```python
from build123d import *

# Parameters (mm, degrees)
EXTRUDE_1_DEPTH     = 20
EXTRUDE_2_DEPTH     = 20
CUT_EXTRUDE_1_DEPTH = 15
SCALE_1_SCALE       = 0.2


with BuildPart() as part:
    # 草圖1 → 填料-伸長1 (new body)
    with BuildSketch(Plane(origin=(0, 0, 0), x_dir=(1, 0, 0), z_dir=(0, 1, 0))):
        Polygon((-5, 5), (-5, -10), (15, -5), (15, 5), align=None)
    extrude(amount=EXTRUDE_1_DEPTH)

    # 草圖1<3> → 填料-伸長2 (add)
    with BuildSketch(Plane(origin=(0, 0, 0), x_dir=(1, 0, 0), z_dir=(0, 1, 0))):
        Polygon((-15, -10), (-5, -10), (-5, 5), (15, 5), (15, 10), (-15, 10), align=None)
    extrude(amount=EXTRUDE_2_DEPTH)

    # 草圖2 → 除料-伸長1 (cut)
    with BuildSketch(Plane.XY.offset(10)):
        Polygon((-5, 20), (15, 5), (15, 20), align=None)
    extrude(amount=-CUT_EXTRUDE_1_DEPTH, mode=Mode.SUBTRACT)


with BuildPart() as part_1:
    # 縮放比例1: scaled about (-2.387387387, 9.02027027, -1.06981982)
    add(part.part.scale(SCALE_1_SCALE).moved(Location((-1.90990991, 7.216216216, -0.855855856))))


solid = part_1.part
```
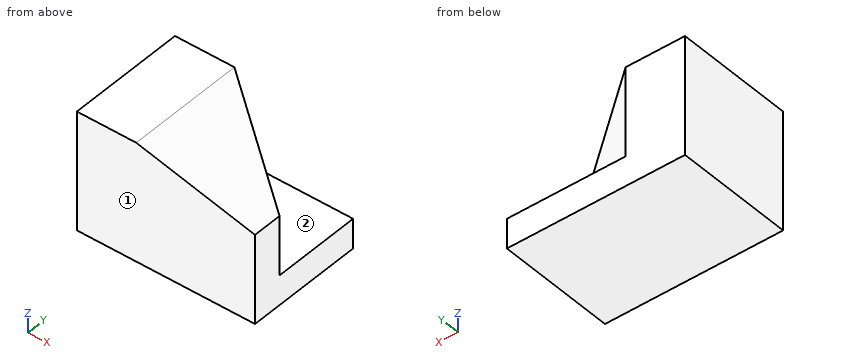
Could you check a few things on this model? Use its own coordinates, in mm. Face numbers are marked on the shaded views. A direction names the side the tool comes from. Coordinates: 2 decimals unless noted, no trailing zeros. Write each loop counter-clockwise with the first axis right and the second up, starting at its lowest first coordinate (ties: lowest second). Pieces come first, ordered by that corner, then holes. Notation, with made-up numbers: (68, 5.25) - (117, 5.25) arc R15 cw to (117, 16.25) - close; hole circle Ø6 at (50, 17.5). An arc over 180 degrees is marked (long way). Use a Markdown table: item, result.
Q1. Imagine slicing it at B-B (z = -0.15). List the corners of the cut face in (x, y) for me.
Geometry check:
| item | result |
|---|---|
| outline | (-4.91, 7.22) - (1.09, 7.22) - (1.09, 8.22) - (-2.91, 11.22) - (-4.91, 11.22) - close |
Q2. Imagine slicing it at A-A (y = 9.9). List the corners of the cut face in (x, z) for me.
Geometry check:
| item | result |
|---|---|
| outline | (-4.91, -2.86) - (1.09, -2.86) - (1.09, -1.86) - (-1.15, -1.86) - (-1.15, 0.71) - (-2.91, 1.14) - (-4.91, 1.14) - close |
Q3. Which directions (+Z, -Z, +X, -X, +Y, -Y) give clear straight access to the entire face, cutting with the end or side of a thin tool? Please do the marked faces 1 and 2.
Geometry check:
| item | result |
|---|---|
| face 1 | +Z, -Z, +X, -X, -Y |
| face 2 | +Z, +X, +Y |
Q4. Please list where these lines run through material, in increasing order: L1, parallel to Z at x = 0.2, y = 9.4; L2, parallel to X at y = 10.45, z = 0.8; L3, parallel to Z at x = -1.5, y = 9.15.
Geometry check:
| item | result |
|---|---|
| L1 | z = -2.86 to -1.86 |
| L2 | x = -4.91 to -1.89 |
| L3 | z = -2.86 to 0.79 |
Q5. Imagine slicing it at D-D (y = 7.5). List the corners of the cut face in (x, z) for me.
Geometry check:
| item | result |
|---|---|
| outline | (-4.91, -2.86) - (1.09, -2.86) - (1.09, 0.14) - (-2.91, 1.14) - (-4.91, 1.14) - close |
Q6. Imagine slicing it at C-C (x = -2.25). List the corners of the cut face in (y, z) for me, and give its area (3 significant figures).
Geometry check:
| item | result |
|---|---|
| outline | (7.22, -2.86) - (11.22, -2.86) - (11.22, -1.86) - (10.72, -1.86) - (10.72, 0.98) - (7.22, 0.98) - close |
| area | 13.9 mm2 |
